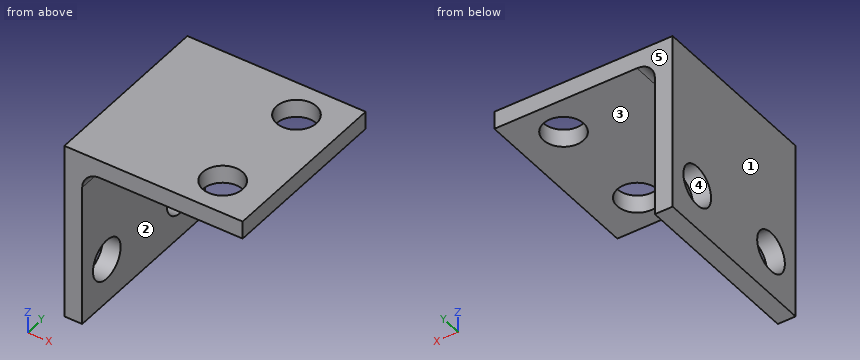
Autodesk Inventor part; units mm, degrees
ref_plane "YZ Plane" through (0, 0, 0) normal (1, 0, 0) x (0, 1, 0)
ref_plane "XZ Plane" through (0, 0, 0) normal (0, 1, 0) x (-1, 0, 0)
ref_plane "XY Plane" through (0, 0, 0) normal (0, 0, 1) x (1, 0, 0)
sketch "Sketch1" plane through (0, 0, 0) normal (0, 0, 1) x (1, 0, 0)
  line L0 (-10, 10) -> (10, 10)
  line L1 (10, 10) -> (10, -10)
  line L2 (10, -10) -> (-10, -10)
  line L3 (-10, -10) -> (-10, 10)
  line L4 (-10, 10) -> (10, -10) construction
  line L5 (10, 10) -> (-10, -10) construction
  point P0 (0, 0)
  dimension "d0" = 20
  dimension "d1" = 20
extrude "Extrusion1" add sketch "Sketch1" against normal blind 2
sketch "Sketch2" plane through (-10, 10, 0) normal (0, 1, 0) x (1, 0, 0)
  line L0 (20, 0) -> (0, 0)
  line L1 (0, 0) -> (2, 0)
  line L2 (2, 0) -> (2, 20)
  line L3 (2, 20) -> (0, 20)
  line L4 (0, 20) -> (0, 0)
  point P0 (10, 0)
  point P1 (2, 0)
  dimension "d4" = 2
  dimension "d5" = 20
extrude "Extrusion2" add sketch "Sketch2" against normal blind 20
fillet "Fillet1" radius 2 1 edges at (-8, 0, -2)
sketch "Sketch4" plane through (0, 0, -2) normal (0, 0, -1) x (-1, 0, 0)
  circle A0 centre (-5, -6) radius 2.25
  circle A1 centre (-5, 6) radius 2.25
  line L0 (-10, -10) -> (6, -10)
  line L1 (6, 10) -> (-10, 10)
  line L2 (-10, 10) -> (-10, -10)
  point P0 (0, 0)
  point P1 (10, -10)
  dimension "d10" = 4.5
  dimension "d11" = 4.5
  dimension "d12" = 4
  dimension "d13" = 4
  dimension "d15" = 5
  dimension "d16" = 5
  dimension "d33" = 12
extrude "Extrusion3" cut sketch "Sketch4" against normal blind 2
sketch "Sketch5" plane through (-8, -10, -20) normal (1, 0, 0) x (0, 0, -1)
  circle A0 centre (-5, 4) radius 2.25
  circle A1 centre (-5, 16) radius 2.25
  line L0 (0, 0) -> (-16, 0)
  line L1 (-16, 20) -> (0, 20)
  line L2 (0, 20) -> (0, 0)
  point P0 (-20, 10)
  dimension "d19" = 4.5
  dimension "d20" = 4.5
  dimension "d21" = 4
  dimension "d23" = 5
  dimension "d24" = 5
  dimension "d38" = 4
extrude "Extrusion4" cut sketch "Sketch5" against normal blind 2
properties part number "CONTROL_MONTEER"
The listing builds one solid part. Answer for the finished solid, in the listing's coordinates (mm). Face numbers are marked on the shaded views. A direction names the side the tool comes from. Coordinates: 2 decimals unless noted, no trailing zeros. Loops run counter-clockwise (first coordinate to the right, second up) from the corner with the lowest first, then second, coordinate; pieces in that order, holes last. Notation, with made-up numbers: (24.25, 72.5) -> (82.25, 72.5) arc R21 ccw to (82.25, 79.5) -> close; hole circle Ø4 at (59.5, 29.25). An arc over 180 degrees is marked (long way). Return JSON: item names as keys, results as strings. Group by question number.
(1) A cutting plane is placed at B-B on z = -15. Write down the section's boundary in (x, y).
(2) Find the intervals of material crossed by probe 1 along Y at (x, z) = (5, -0.6); probe 2 along Z at (x, y) = (1.5, -1); probe 3 along X at (y, z) = (-4.5, -5.5), in increasing order. Write a range as from..to.
(3) Determine the mould class of the marked faces 3, 4 and 5 for opening direction Z: released by +Z, released by -Z, zero draft, split by the parting line, or undercut.
(4) Which of the six approach directions +Z, -Z, +X, -X, +Y, -Y give full straight-line access (tool end or side, diameter ignored) to the marked faces 1 and 2?
(5) A cutting plane is placed at C-C on x = 5. Write down the section's boundary in (y, z), and give its area (3 significant figures).
(6) Given pin 1 Ø8 at (y, z) = (-4, -15) entering from +X; pin 2 Ø4 at (x, y) = (-0.5, 7.5) entering from -Z; pin 3 Ø4 at (x, y) = (-5, -4) entering from -Z, each flat-ended and moving along its own axis, determine where each tip first touches the part or whether it passes through.
(7) A cutting plane is placed at D-D on y = 2. Write down the section's boundary in (x, z).
(8) A cutting plane is placed at A-A on y = 6. Write down the section's boundary in (x, z).
The answers:
{
 "1": {"outline": "(-10, -10) -> (-8, -10) -> (-8, -8.25) -> (-10, -8.25) -> close; (-10, -3.75) -> (-8, -3.75) -> (-8, 3.75) -> (-10, 3.75) -> close; (-10, 8.25) -> (-8, 8.25) -> (-8, 10) -> (-10, 10) -> close"},
 "2": {"probe 1": "y = -10..-8.25, -3.75..3.75, 8.25..10", "probe 2": "z = -2..0", "probe 3": "x = -10..-8"},
 "3": {"face 3": "released by -Z", "face 4": "undercut", "face 5": "zero draft"},
 "4": {"face 1": "+Z, -Z, -X, +Y, -Y", "face 2": "-Z, +X, +Y, -Y"},
 "5": {"outline": "(-10, -2) -> (-8.25, -2) -> (-8.25, 0) -> (-10, 0) -> close; (-3.75, -2) -> (3.75, -2) -> (3.75, 0) -> (-3.75, 0) -> close; (8.25, -2) -> (10, -2) -> (10, 0) -> (8.25, 0) -> close", "area": "22.0 mm^2"},
 "6": {"pin 1": "stops at x = -8", "pin 2": "stops at z = -2", "pin 3": "stops at z = -2.27"},
 "7": {"outline": "(-10, -20) -> (-8, -20) -> (-8, -4) arc R2 cw to (-6, -2) -> (10, -2) -> (10, 0) -> (-10, 0) -> close"},
 "8": {"outline": "(-10, -20) -> (-8, -20) -> (-8, -17.25) -> (-10, -17.25) -> close; (-10, -12.75) -> (-8, -12.75) -> (-8, -4) arc R2 cw to (-6, -2) -> (2.75, -2) -> (2.75, 0) -> (-10, 0) -> close; (7.25, -2) -> (10, -2) -> (10, 0) -> (7.25, 0) -> close"}
}
